from build123d import *

# Parameters (mm, degrees)
CROQUIS1_W              = 77
CROQUIS1_H              = 45
SALIENTE_EXTRUIR1_DEPTH = 3
CORTAR_EXTRUIR1_REACH   = 5
CROQUIS2_R              = 1.6
CROQUIS2_W              = 17
CROQUIS2_H              = 12.6
CROQUIS2_W_2            = 10.65
CROQUIS2_H_2            = 12
CROQUIS2_W_3            = 9.15
CROQUIS2_W_4            = 15.1
CROQUIS2_H_3            = 7.1


with BuildPart() as part:
    # Croquis1 → Saliente-Extruir1 (new body)
    with BuildSketch(Plane.XY):
        with Locations((38.5, 22.5)):
            Rectangle(CROQUIS1_W, CROQUIS1_H)
    extrude(amount=SALIENTE_EXTRUIR1_DEPTH)

    # Croquis2 → Cortar-Extruir1 (cut, up to next)
    with BuildSketch(Plane.XY.offset(3), mode=Mode.PRIVATE) as cortar_extruir1_sk1:
        with Locations((3.75, 40)):
            Circle(CROQUIS2_R)
    cortar_extruir1_tool1 = extrude(cortar_extruir1_sk1.sketch, amount=-CORTAR_EXTRUIR1_REACH, mode=Mode.PRIVATE) & part.part
    add(cortar_extruir1_tool1.solids().sort_by_distance((3.75, 40, 3))[0], mode=Mode.SUBTRACT)
    # Croquis2 → Cortar-Extruir1 (cut, up to next)
    with BuildSketch(Plane.XY.offset(3), mode=Mode.PRIVATE) as cortar_extruir1_sk2:
        with Locations((3.75, 5)):
            Circle(CROQUIS2_R)
    cortar_extruir1_tool2 = extrude(cortar_extruir1_sk2.sketch, amount=-CORTAR_EXTRUIR1_REACH, mode=Mode.PRIVATE) & part.part
    add(cortar_extruir1_tool2.solids().sort_by_distance((3.75, 5, 3))[0], mode=Mode.SUBTRACT)
    # Croquis2 → Cortar-Extruir1 (cut, up to next)
    with BuildSketch(Plane.XY.offset(3), mode=Mode.PRIVATE) as cortar_extruir1_sk3:
        with Locations((73.25, 5)):
            Circle(CROQUIS2_R)
    cortar_extruir1_tool3 = extrude(cortar_extruir1_sk3.sketch, amount=-CORTAR_EXTRUIR1_REACH, mode=Mode.PRIVATE) & part.part
    add(cortar_extruir1_tool3.solids().sort_by_distance((73.25, 5, 3))[0], mode=Mode.SUBTRACT)
    # Croquis2 → Cortar-Extruir1 (cut, up to next)
    with BuildSketch(Plane.XY.offset(3), mode=Mode.PRIVATE) as cortar_extruir1_sk4:
        with Locations((73.25, 40)):
            Circle(CROQUIS2_R)
    cortar_extruir1_tool4 = extrude(cortar_extruir1_sk4.sketch, amount=-CORTAR_EXTRUIR1_REACH, mode=Mode.PRIVATE) & part.part
    add(cortar_extruir1_tool4.solids().sort_by_distance((73.25, 40, 3))[0], mode=Mode.SUBTRACT)
    # Croquis2 → Cortar-Extruir1 (cut, up to next)
    with BuildSketch(Plane.XY.offset(3), mode=Mode.PRIVATE) as cortar_extruir1_sk5:
        with Locations((33.45, 21.5)):
            Circle(CROQUIS2_R)
    cortar_extruir1_tool5 = extrude(cortar_extruir1_sk5.sketch, amount=-CORTAR_EXTRUIR1_REACH, mode=Mode.PRIVATE) & part.part
    add(cortar_extruir1_tool5.solids().sort_by_distance((33.45, 21.5, 3))[0], mode=Mode.SUBTRACT)
    # Croquis2 → Cortar-Extruir1 (cut, up to next)
    with BuildSketch(Plane.XY.offset(3), mode=Mode.PRIVATE) as cortar_extruir1_sk6:
        with Locations((33.45, 6)):
            Circle(CROQUIS2_R)
    cortar_extruir1_tool6 = extrude(cortar_extruir1_sk6.sketch, amount=-CORTAR_EXTRUIR1_REACH, mode=Mode.PRIVATE) & part.part
    add(cortar_extruir1_tool6.solids().sort_by_distance((33.45, 6, 3))[0], mode=Mode.SUBTRACT)
    # Croquis2 → Cortar-Extruir1 (cut, up to next)
    with BuildSketch(Plane.XY.offset(3), mode=Mode.PRIVATE) as cortar_extruir1_sk7:
        with Locations((62.35, 21.5)):
            Circle(CROQUIS2_R)
    cortar_extruir1_tool7 = extrude(cortar_extruir1_sk7.sketch, amount=-CORTAR_EXTRUIR1_REACH, mode=Mode.PRIVATE) & part.part
    add(cortar_extruir1_tool7.solids().sort_by_distance((62.35, 21.5, 3))[0], mode=Mode.SUBTRACT)
    # Croquis2 → Cortar-Extruir1 (cut, up to next)
    with BuildSketch(Plane.XY.offset(3), mode=Mode.PRIVATE) as cortar_extruir1_sk8:
        with Locations((62.35, 6)):
            Circle(CROQUIS2_R)
    cortar_extruir1_tool8 = extrude(cortar_extruir1_sk8.sketch, amount=-CORTAR_EXTRUIR1_REACH, mode=Mode.PRIVATE) & part.part
    add(cortar_extruir1_tool8.solids().sort_by_distance((62.35, 6, 3))[0], mode=Mode.SUBTRACT)
    # Croquis2 → Cortar-Extruir1 (cut, up to next)
    with BuildSketch(Plane.XY.offset(3), mode=Mode.PRIVATE) as cortar_extruir1_sk9:
        with Locations((17.5, 17.5)):
            Rectangle(CROQUIS2_W, CROQUIS2_H)
    cortar_extruir1_tool9 = extrude(cortar_extruir1_sk9.sketch, amount=-CORTAR_EXTRUIR1_REACH, mode=Mode.PRIVATE) & part.part
    add(cortar_extruir1_tool9.solids().sort_by_distance((17.5, 17.5, 3))[0], mode=Mode.SUBTRACT)
    # Croquis2 → Cortar-Extruir1 (cut, up to next)
    with BuildSketch(Plane.XY.offset(3), mode=Mode.PRIVATE) as cortar_extruir1_sk10:
        with Locations((28.975, 35.3)):
            Rectangle(CROQUIS2_W_2, CROQUIS2_H_2)
    cortar_extruir1_tool10 = extrude(cortar_extruir1_sk10.sketch, amount=-CORTAR_EXTRUIR1_REACH, mode=Mode.PRIVATE) & part.part
    add(cortar_extruir1_tool10.solids().sort_by_distance((28.975, 35.3, 3))[0], mode=Mode.SUBTRACT)
    # Croquis2 → Cortar-Extruir1 (cut, up to next)
    with BuildSketch(Plane.XY.offset(3), mode=Mode.PRIVATE) as cortar_extruir1_sk11:
        with Locations((48.775, 35.3)):
            Rectangle(CROQUIS2_W_3, CROQUIS2_H_2)
    cortar_extruir1_tool11 = extrude(cortar_extruir1_sk11.sketch, amount=-CORTAR_EXTRUIR1_REACH, mode=Mode.PRIVATE) & part.part
    add(cortar_extruir1_tool11.solids().sort_by_distance((48.775, 35.3, 3))[0], mode=Mode.SUBTRACT)
    # Croquis2 → Cortar-Extruir1 (cut, up to next)
    with BuildSketch(Plane.XY.offset(3), mode=Mode.PRIVATE) as cortar_extruir1_sk12:
        with Locations((47.9, 21.5)):
            Rectangle(CROQUIS2_W_4, CROQUIS2_H_3)
    cortar_extruir1_tool12 = extrude(cortar_extruir1_sk12.sketch, amount=-CORTAR_EXTRUIR1_REACH, mode=Mode.PRIVATE) & part.part
    add(cortar_extruir1_tool12.solids().sort_by_distance((47.9, 21.5, 3))[0], mode=Mode.SUBTRACT)
    # Croquis2 → Cortar-Extruir1 (cut, up to next)
    with BuildSketch(Plane.XY.offset(3), mode=Mode.PRIVATE) as cortar_extruir1_sk13:
        with Locations((47.9, 6)):
            Rectangle(CROQUIS2_W_4, CROQUIS2_H_3)
    cortar_extruir1_tool13 = extrude(cortar_extruir1_sk13.sketch, amount=-CORTAR_EXTRUIR1_REACH, mode=Mode.PRIVATE) & part.part
    add(cortar_extruir1_tool13.solids().sort_by_distance((47.9, 6, 3))[0], mode=Mode.SUBTRACT)


solid = part.part
Design review of the part built by this model. Coordinates are the model's own, in mm. A direction names the side the tool comes from. Round coordinates to 2 decimals unless told otherwise and drop trailing zeros. Order: outer loops, then holes, each group sorted by start corner. A loop starts at its lowest first (then second) coordinate and runs counter-clockwise, first axis right, second up. Notation, with made-up numbers: M -21.75,69.25 L -13.75,69.25 A33 ccw -13.75,104.25 Z; hole C 6,32 d4. An arc over 180 degrees is marked long. Answer as CSV lines item,"result". Start each with the question number.
1) Wall thickness on line 1 along Y through (x, z) = (44.5, 1.6); line 2 along Y through (x, z) = (54.5, 0.25); line 3 along Y through (x, z) = (62.35, 1): over which ranges is each line inside the solid? List them lowest first. Write a range as [from, to].
2) Add section A-A (x = 3.75). Give the boundary of the cut face in (y, z).
3) The part is to be moulded in two halves that separate along X. For faces 3 (the face through (38, 45, 1)), 4 (the face through (40.35, 21, 2)), 5 (the face through (0, 22, 1)), say which applies: +X half, -X half, draft (parallel to the pull), parting line (faces both ways), or undercut.
4) Tool access review of faces 1 (the face through (48, 25.05, 2)), 2 (the face through (77, 22, 1)): name each direction out of +Z, -Z, +X, -X, +Y, -Y from which nothing blocks a thin tool from reaching the whole face with its end or side.
5) Add section D-D (x = 51.5). Give the boundary of the cut face in (y, z), then the cut area to 3 significant figures.
6) For pin 1 Ø3 at (x, y) = (62.35, 6) entering from -Z, flat-tipped, find the tip position at first contact; note if it passes through.
7) Add section C-C (z = 1.45). Give the number of separate pieces and of enclosed holes in the cut face, then the cut area to 3 significant figures.
8) Add section B-B (y = 19). Give the boundary of the cut face in (x, z).
Resolved:
1,line 1,"[0, 2.45], [9.55, 17.95], [25.05, 29.3], [41.3, 45]"
1,line 2,"[0, 2.45], [9.55, 17.95], [25.05, 45]"
1,line 3,"[0, 4.4], [7.6, 19.9], [23.1, 45]"
2,outline,"M 0,0 L 3.4,0 L 3.4,3 L 0,3 Z; M 6.6,0 L 38.4,0 L 38.4,3 L 6.6,3 Z; M 41.6,0 L 45,0 L 45,3 L 41.6,3 Z"
3,face 3,"draft"
3,face 4,"undercut"
3,face 5,"-X half"
4,face 1,"+Z, -Z"
4,face 2,"+Z, -Z, +X, +Y, -Y"
5,outline,"M 0,0 L 2.45,0 L 2.45,3 L 0,3 Z; M 9.55,0 L 17.95,0 L 17.95,3 L 9.55,3 Z; M 25.05,0 L 29.3,0 L 29.3,3 L 25.05,3 Z; M 41.3,0 L 45,0 L 45,3 L 41.3,3 Z"
5,area,"56.4 mm^2"
6,pin 1,"through"
7,separate pieces,"1"
7,enclosed holes,"13"
7,area,"2,730 mm^2"
8,outline,"M 0,0 L 9,0 L 9,3 L 0,3 Z; M 26,0 L 40.35,0 L 40.35,3 L 26,3 Z; M 55.45,0 L 77,0 L 77,3 L 55.45,3 Z"
